from build123d import *

# Parameters (mm, degrees)
SKETCH_1_R               = 31
EXTRUDE_1_DEPTH          = 30
CUT_EXTRUDE_3_DEPTH      = 51.467811524
CUT_EXTRUDE_3_DEPTH_BACK = 51.467811524
SKETCH_5_R               = 16
SKETCH_6_R               = 29
CUT_EXTRUDE_4_DEPTH      = 26
HOLE_WIZARD_M2_5_1_D     = 2.05


with BuildPart() as part:
    # 草图1 → 凸台-拉伸1 (new body)
    with BuildSketch(Plane(origin=(0, 0, 0), x_dir=(1, 0, 0), z_dir=(0, 1, 0))):
        with Locations(Location((0, 0, 0), (0, 0, 270))):
            Circle(SKETCH_1_R)
    extrude(amount=EXTRUDE_1_DEPTH)

    # 草图5 → 切除-拉伸3 (cut, two sides: drawn at the far end of the back side and taken through both)
    with BuildSketch(Plane(origin=(0, 5, 0), x_dir=(-1, 0, 0), z_dir=(0, -1, 0)).offset(-CUT_EXTRUDE_3_DEPTH_BACK)):
        with Locations(Location((0, 0, 0), (0, 0, 90))):
            Circle(SKETCH_5_R)
    extrude(amount=CUT_EXTRUDE_3_DEPTH + CUT_EXTRUDE_3_DEPTH_BACK, mode=Mode.SUBTRACT)

    # 草图6 → 切除-拉伸4 (cut)
    with BuildSketch(Plane(origin=(0, 30, 0), x_dir=(1, 0, 0), z_dir=(0, 1, 0))):
        with Locations(Location((0, 0, 0), (0, 0, 270))):
            Circle(SKETCH_6_R)
    extrude(amount=-CUT_EXTRUDE_4_DEPTH, mode=Mode.SUBTRACT)

    # M2.5 螺纹孔1 (through all)
    with Locations(Plane(origin=(0, 4, 0), x_dir=(1, 0, 0), z_dir=(0, 1, 0))):
        with Locations((-16.455, 9.5), (16.455, 9.5), (16.455, -9.5), (-16.455, -9.5)):
            Hole(HOLE_WIZARD_M2_5_1_D / 2)


solid = part.part
Build history of the part. All positions in model axes, mm. A direction names the side the tool comes from. Round coordinates to 2 decimals unless told otherwise and drop trailing zeros. Write each loop counter-clockwise with the first axis right and the second up, starting at its lowest first coordinate (ties: lowest second). Pieces come first, ordered by that corner, then holes. Notation, with made-up numbers: M 70,54 L 97,54 A15 ccw 97,76 Z; hole C 53.5,4.25 d3. An arc over 180 degrees is marked long. Answer in a Markdown table with one row per item.
1. Mould opens along X. For faces 1 (the face through (30.736, 14.79, -4.036)), 2 (the face through (15.48, 1.97, 9.19)), 3 (the face through (-15.43, 1.97, -9.55)), 4 (the face through (-21, 30, 21)) say: +X half, -X half, draft (parallel to the pull), parting line (faces both ways), or undercut.
Geometry check:
| item | result |
|---|---|
| face 1 | parting line |
| face 2 | undercut |
| face 3 | undercut |
| face 4 | draft |
2. Saw through at D-D (z = -9.5). List the corners of the cut face in (x, y).
Geometry check:
| item | result |
|---|---|
| outline | M -29.51,0 L -17.48,0 L -17.48,4 L -27.4,4 L -27.4,30 L -29.51,30 Z; M -15.43,0 L -12.87,0 L -12.87,4 L -15.43,4 Z; M 12.87,0 L 15.43,0 L 15.43,4 L 12.87,4 Z; M 17.48,0 L 29.51,0 L 29.51,30 L 27.4,30 L 27.4,4 L 17.48,4 Z |
3. Saw through at C-C (y = 27.75). List the corners of the cut face in (x, z).
Geometry check:
| item | result |
|---|---|
| outline | C 0,0 d62; hole C 0,0 d58 |
4. Probe L1, parallel to X at y = 0.8, z = 0; L2, parallel to X at y = 17.5, z = 0; L3, parallel to Y at x = 9, z = -18.5. List the from-to ranges inside material, lowest first. Write a range as [from, to].
Geometry check:
| item | result |
|---|---|
| L1 | [-31, -16], [16, 31] |
| L2 | [-31, -29], [29, 31] |
| L3 | [0, 4] |
5. Which spindle directions (+Z, -Z, +X, -X, +Y, -Y) get a long thin tool onto all of the face, cutting with end or side? Do faces 5 (the face through (-11.107, 17.182, 26.789)), 6 (the face through (15.48, 1.97, -9.81)). Say none if no direction does.
Geometry check:
| item | result |
|---|---|
| face 5 | +Y |
| face 6 | +Y, -Y |
6. Saw through at B-B (z = 0). List the corners of the cut face in (x, y), and give its area (3 significant figures).
Geometry check:
| item | result |
|---|---|
| outline | M -31,0 L -16,0 L -16,4 L -29,4 L -29,30 L -31,30 Z; M 16,0 L 31,0 L 31,30 L 29,30 L 29,4 L 16,4 Z |
| area | 224 mm2 |
7. Flat gauge pins, fed straight in: P1, Ø6, axis at y = 19.5, z = 15.5, coming from the +X side; P2, Ø2.5, axis at x = -16.455, z = -9.5, coming from the +Y side; P3, Ø2, axis at y = 23.5, z = 13.5, coming from the -X side. Where does each tip first touch, or does it go through?
Geometry check:
| item | result |
|---|---|
| P1 | x = 28.37 |
| P2 | y = 4 |
| P3 | x = -28.37 |
8. Saw through at A-A (x = 0). List the corners of the cut face in (y, z), and give its area (3 significant figures).
Geometry check:
| item | result |
|---|---|
| outline | M 0,-31 L 30,-31 L 30,-29 L 4,-29 L 4,-16 L 0,-16 Z; M 0,16 L 4,16 L 4,29 L 30,29 L 30,31 L 0,31 Z |
| area | 224 mm2 |
